For this review, take the finished solid that the model builds, in its own axes (mm). A direction names the side the tool comes from. Give positions to 0.01 mm unless a question says otherwise; leave off trailing zeros. Write each loop counter-clockwise with the first axis right and the second up, starting at its lowest first coordinate (ties: lowest second). Pieces come first, ordered by that corner, then holes.
Q1. For line 1 (X direction, y = 0, z = 13.75); line 2 (X direction, y = -28, z = 12.5); line 3 (Y direction, x = 16, z = 56.5), list the stretches that pass through material, from the lowest coordinate up.
Q2. Insertion check: P1, Ø1.5, axis at y = 7, z = 74.5, coming from the -X side; P2, Ø10, axis at x = -24, z = 61.5, coming from the +Y side; P3, Ø3, axis at y = 27, z = 9, coming from the +X side; P4, Ø10, axis at x = 15, y = 26.5, coming from the +Z side. Each pin has a flat end and moves straight along its axis. Give the tip position at first contact, or say it passes through.
Q3. Mouldability with a two-part tool opening along Z and no side actions: class faces 4 (the cylindrical face through (-1.64, -23.66, 18.9)), 5 (the cylindrical face through (0, -29, 81)), 6 (the cylindrical face through (-23.7, -1.64, 24.1)) as released by +Z, released by -Z, zero draft, split by the parting line, or undercut.
Q4. We need section A-A (y = -26). Write out the cut boundary in (x, z), then the cut area to 3 significant figures.
Q5. We need section B-B (x = -28). Write out the cut boundary in (y, z), then the cut area to 3 significant figures.
Q6. Machinability: for faces 1 (the flat face through (27, -5, 11)), 2 (the cylindrical face through (3.64, 23.52, 18.9)), 3 (the flat face through (5, 27, 11)), which of the approach directions +Z, -Z, +X, -X, +Y, -Y give a long, thin tool a straight path to every point of the face, cutting with its end or side? Answer none if there is none.
Q7. We need section D-D (y = 28). Write out the cut boundary in (x, z), then the cut area to 3 significant figures.
Q8. We need section C-C (z = 11). Give the number of separate pieces and of enclosed holes in the cut face, then the cut area to 3 significant figures.
```python
from build123d import *

# Parameters (mm, degrees)
CYLINDER019_R              = 1
CYLINDER019_DEPTH          = 10
BOX007_W                   = 10
BOX007_H                   = 10
BOX007_DEPTH               = 10
CHAMFER004_SIZE            = 3
CHAMFER004_PLACEMENT_ANGLE = -90
CYLINDER015_R              = 1
CYLINDER015_DEPTH          = 10
BOX002_W                   = 10
BOX002_H                   = 10
BOX002_DEPTH               = 10
CHAMFER_SIZE               = 3
CYLINDER017_R              = 1
CYLINDER017_DEPTH          = 10
BOX005_W                   = 10
BOX005_H                   = 10
BOX005_DEPTH               = 10
CHAMFER002_SIZE            = 3
CYLINDER018_R              = 1
CYLINDER018_DEPTH          = 10
BOX006_W                   = 10
BOX006_H                   = 10
BOX006_DEPTH               = 10
CHAMFER003_SIZE            = 3
CHAMFER003_PLACEMENT_ANGLE = 90
CYLINDER020_R              = 1
CYLINDER020_DEPTH          = 10
BOX008_W                   = 10
BOX008_H                   = 10
BOX008_DEPTH               = 10
CHAMFER005_SIZE            = 3
CHAMFER005_PLACEMENT_ANGLE = 180
CYLINDER_R                 = 1
CYLINDER_DEPTH             = 10
BOX004_W                   = 10
BOX004_H                   = 10
BOX004_DEPTH               = 10
CHAMFER001_SIZE            = 3
CHAMFER001_PLACEMENT_ANGLE = 180
BOX001_W                   = 7
BOX001_H                   = 120
BOX001_DEPTH               = 7
BOX001_PLACEMENT_ANGLE     = 90
FILLET_R                   = 3
BOX_W                      = 7
BOX_H                      = 120
BOX_DEPTH                  = 7
FILLET001_R                = 3
CYLINDER009_R              = 22.5
CYLINDER009_DEPTH          = 80
CYLINDER008_R              = 25
CYLINDER008_DEPTH          = 80


with BuildPart() as cylindre020:
    # Cylinder019 → Cylinder019 (new body)
    with BuildSketch(Plane(origin=(5, 5, 0), x_dir=(1, 0, 0), z_dir=(0, 0, 1))):
        Circle(CYLINDER019_R)
    extrude(amount=CYLINDER019_DEPTH)


with BuildPart() as chamfer004:
    # Box007 → Box007 (new body)
    with BuildSketch(Plane.XY):
        with Locations((5, 5)):
            Rectangle(BOX007_W, BOX007_H)
    extrude(amount=BOX007_DEPTH)

    # Cut018: cut Cylindre020
    add(cylindre020.part, mode=Mode.SUBTRACT)


with BuildPart() as chamfer004_1:
    # Cut018 placement: moved
    add(chamfer004.part.moved(Location((-5, 48, 70))))

    # Chamfer004
    chamfer004_edges = [chamfer004_1.edges().sort_by_distance(p)[0] for p in [
        (-5, 58, 75),
        (5, 58, 75),
    ]]
    chamfer(chamfer004_edges, length=CHAMFER004_SIZE)


with BuildPart() as chamfer004_2:
    # Chamfer004 placement: moved
    add(chamfer004_1.part.moved(Location((-25, 0, -70))).rotate(Axis((-25, 0, -70), (0, 0, 1)), CHAMFER004_PLACEMENT_ANGLE))


with BuildPart() as cylindre:
    # Cylinder015 → Cylinder015 (new body)
    with BuildSketch(Plane(origin=(5, 5, 0), x_dir=(1, 0, 0), z_dir=(0, 0, 1))):
        Circle(CYLINDER015_R)
    extrude(amount=CYLINDER015_DEPTH)


with BuildPart() as chamfer_body:
    # Box002 → Box002 (new body)
    with BuildSketch(Plane.XY):
        with Locations((5, 5)):
            Rectangle(BOX002_W, BOX002_H)
    extrude(amount=BOX002_DEPTH)

    # Cut014: cut Cylindre
    add(cylindre.part, mode=Mode.SUBTRACT)


with BuildPart() as chamfer_body_1:
    # Cut014 placement: moved
    add(chamfer_body.part.moved(Location((-5, 48, 70))))

    # Chamfer
    chamfer_edges = [chamfer_body_1.edges().sort_by_distance(p)[0] for p in [
        (-5, 58, 75),
        (5, 58, 75),
    ]]
    chamfer(chamfer_edges, length=CHAMFER_SIZE)


with BuildPart() as chamfer_body_2:
    # Chamfer placement: moved
    add(chamfer_body_1.part.moved(Location((0, -25, 0))))


with BuildPart() as cylindre018:
    # Cylinder017 → Cylinder017 (new body)
    with BuildSketch(Plane(origin=(5, 5, 0), x_dir=(1, 0, 0), z_dir=(0, 0, 1))):
        Circle(CYLINDER017_R)
    extrude(amount=CYLINDER017_DEPTH)


with BuildPart() as chamfer002:
    # Box005 → Box005 (new body)
    with BuildSketch(Plane.XY):
        with Locations((5, 5)):
            Rectangle(BOX005_W, BOX005_H)
    extrude(amount=BOX005_DEPTH)

    # Cut016: cut Cylindre018
    add(cylindre018.part, mode=Mode.SUBTRACT)


with BuildPart() as chamfer002_1:
    # Cut016 placement: moved
    add(chamfer002.part.moved(Location((-5, 48, 70))))

    # Chamfer002
    chamfer002_edges = [chamfer002_1.edges().sort_by_distance(p)[0] for p in [
        (-5, 58, 75),
        (5, 58, 75),
    ]]
    chamfer(chamfer002_edges, length=CHAMFER002_SIZE)


with BuildPart() as chamfer002_2:
    # Chamfer002 placement: moved
    add(chamfer002_1.part.moved(Location((0, -25, -70))))


with BuildPart() as cylindre019:
    # Cylinder018 → Cylinder018 (new body)
    with BuildSketch(Plane(origin=(5, 5, 0), x_dir=(1, 0, 0), z_dir=(0, 0, 1))):
        Circle(CYLINDER018_R)
    extrude(amount=CYLINDER018_DEPTH)


with BuildPart() as chamfer003:
    # Box006 → Box006 (new body)
    with BuildSketch(Plane.XY):
        with Locations((5, 5)):
            Rectangle(BOX006_W, BOX006_H)
    extrude(amount=BOX006_DEPTH)

    # Cut017: cut Cylindre019
    add(cylindre019.part, mode=Mode.SUBTRACT)


with BuildPart() as chamfer003_1:
    # Cut017 placement: moved
    add(chamfer003.part.moved(Location((-5, 48, 70))))

    # Chamfer003
    chamfer003_edges = [chamfer003_1.edges().sort_by_distance(p)[0] for p in [
        (-5, 58, 75),
        (5, 58, 75),
    ]]
    chamfer(chamfer003_edges, length=CHAMFER003_SIZE)


with BuildPart() as chamfer003_2:
    # Chamfer003 placement: moved
    add(chamfer003_1.part.moved(Location((25, 1.5, -70))).rotate(Axis((25, 1.5, -70), (0, 0, 1)), CHAMFER003_PLACEMENT_ANGLE))


with BuildPart() as cylindre021:
    # Cylinder020 → Cylinder020 (new body)
    with BuildSketch(Plane(origin=(5, 5, 0), x_dir=(1, 0, 0), z_dir=(0, 0, 1))):
        Circle(CYLINDER020_R)
    extrude(amount=CYLINDER020_DEPTH)


with BuildPart() as chamfer005:
    # Box008 → Box008 (new body)
    with BuildSketch(Plane.XY):
        with Locations((5, 5)):
            Rectangle(BOX008_W, BOX008_H)
    extrude(amount=BOX008_DEPTH)

    # Cut019: cut Cylindre021
    add(cylindre021.part, mode=Mode.SUBTRACT)


with BuildPart() as chamfer005_1:
    # Cut019 placement: moved
    add(chamfer005.part.moved(Location((-5, 48, 70))))

    # Chamfer005
    chamfer005_edges = [chamfer005_1.edges().sort_by_distance(p)[0] for p in [
        (-5, 58, 75),
        (5, 58, 75),
    ]]
    chamfer(chamfer005_edges, length=CHAMFER005_SIZE)


with BuildPart() as chamfer005_2:
    # Chamfer005 placement: moved
    add(chamfer005_1.part.moved(Location((0, 25, -70))).rotate(Axis((0, 25, -70), (0, 0, 1)), CHAMFER005_PLACEMENT_ANGLE))


with BuildPart() as cylindre017:
    # Cylinder → Cylinder (new body)
    with BuildSketch(Plane(origin=(5, 5, 0), x_dir=(1, 0, 0), z_dir=(0, 0, 1))):
        Circle(CYLINDER_R)
    extrude(amount=CYLINDER_DEPTH)


with BuildPart() as obj1:
    # Box004 → Box004 (new body)
    with BuildSketch(Plane.XY):
        with Locations((5, 5)):
            Rectangle(BOX004_W, BOX004_H)
    extrude(amount=BOX004_DEPTH)

    # Cut015: cut Cylindre017
    add(cylindre017.part, mode=Mode.SUBTRACT)


with BuildPart() as obj1_1:
    # Cut015 placement: moved
    add(obj1.part.moved(Location((-5, 48, 70))))

    # Chamfer001
    chamfer001_edges = [obj1_1.edges().sort_by_distance(p)[0] for p in [
        (-5, 58, 75),
        (5, 58, 75),
    ]]
    chamfer(chamfer001_edges, length=CHAMFER001_SIZE)


with BuildPart() as obj1_2:
    # Chamfer001 placement: moved
    add(obj1_1.part.moved(Location((0, 25, 0))).rotate(Axis((0, 25, 0), (0, 0, 1)), CHAMFER001_PLACEMENT_ANGLE))

    # Fusion: union Chamfer004, Chamfer body, Chamfer002, Chamfer003, Chamfer005
    add(chamfer004_2.part)
    add(chamfer_body_2.part)
    add(chamfer002_2.part)
    add(chamfer003_2.part)
    add(chamfer005_2.part)


with BuildPart() as fillet_body:
    # Box001 → Box001 (new body)
    with BuildSketch(Plane.XY):
        with Locations((3.5, 60)):
            Rectangle(BOX001_W, BOX001_H)
    extrude(amount=BOX001_DEPTH)


with BuildPart() as fillet_body_1:
    # Box001 placement: moved
    add(fillet_body.part.moved(Location((60, -2.5, 12))).rotate(Axis((60, -2.5, 12), (0, 0, 1)), BOX001_PLACEMENT_ANGLE))

    # Fillet
    fillet_edges = [fillet_body_1.edges().sort_by_distance(p)[0] for p in [
        (0, -2.5, 19),
        (0, -2.5, 12),
        (0, 4.5, 19),
        (0, 4.5, 12),
    ]]
    fillet(fillet_edges, radius=FILLET_R)


with BuildPart() as fillet001:
    # Box → Box (new body)
    with BuildSketch(Plane(origin=(-2.5, -60, 12), x_dir=(1, 0, 0), z_dir=(0, 0, 1))):
        with Locations((3.5, 60)):
            Rectangle(BOX_W, BOX_H)
    extrude(amount=BOX_DEPTH)

    # Fillet001
    fillet001_edges = [fillet001.edges().sort_by_distance(p)[0] for p in [
        (-2.5, 0, 19),
        (-2.5, 0, 12),
        (4.5, 0, 19),
        (4.5, 0, 12),
    ]]
    fillet(fillet001_edges, radius=FILLET001_R)


with BuildPart() as cylindre009:
    # Cylinder009 → Cylinder009 (new body)
    with BuildSketch(Plane.XY):
        Circle(CYLINDER009_R)
    extrude(amount=CYLINDER009_DEPTH)


with BuildPart() as obj2:
    # Cylinder008 → Cylinder008 (new body)
    with BuildSketch(Plane.XY):
        Circle(CYLINDER008_R)
    extrude(amount=CYLINDER008_DEPTH)

    # Cut008: cut Cylindre009
    add(cylindre009.part, mode=Mode.SUBTRACT)

    # Cut: cut Fillet001
    add(fillet001.part, mode=Mode.SUBTRACT)

    # Cut009: cut Fillet body
    add(fillet_body_1.part, mode=Mode.SUBTRACT)

    # Fusion001: union obj1
    add(obj1_2.part)


with BuildPart() as obj2_1:
    # Fusion001 placement: moved
    add(obj2.part.moved(Location((0, 0, 6))))


solid = obj2_1.part
```
Computed:
1. line 1: x = -33 to -22.5, 22.5 to 27, 29 to 33
1. line 2: x = -5 to -1, 1 to 5
1. line 3: y = -19.21 to -15.82, 15.82 to 19.21
2. P1: stops at x = -24.21
2. P2: stops at y = 16.25
2. P3: stops at x = 5
2. P4: passes through
3. face 4: undercut
3. face 5: zero draft
3. face 6: undercut
4. outline: (-5, 6) - (5, 6) - (5, 16) - (-5, 16) - close; (-5, 76) - (5, 76) - (5, 86) - (-5, 86) - close
4. area: 200 mm2
5. outline: (-3.5, 6) - (0.5, 6) - (0.5, 16) - (-3.5, 16) - close; (2.5, 6) - (6.5, 6) - (6.5, 16) - (2.5, 16) - close
5. area: 80.0 mm2
6. face 1: +Z, -Z, +X, -Y
6. face 2: +Y, -Y
6. face 3: +Z, -Z, +X, +Y
7. outline: (-5, 6) - (-1, 6) - (-1, 16) - (-5, 16) - close; (-5, 76) - (-1, 76) - (-1, 86) - (-5, 86) - close; (1, 6) - (5, 6) - (5, 16) - (1, 16) - close; (1, 76) - (5, 76) - (5, 86) - (1, 86) - close
7. area: 160 mm2
8. separate pieces: 1
8. enclosed holes: 5
8. area: 652 mm2
